The drawing under review shows one solid part. Ordinate dimensions are in mm from its lowest x, y, z. A direction names the side the tool comes from. Round coordinates to 2 decimals unless told otherwise and drop trailing zeros. Order: outer loops, then holes, each group sorted by start corner. A loop starts at its lowest first (then second) coordinate and runs counter-clockwise, first axis right, second up. Notation, with made-up numbers: (88, 43.5) - (124, 43.5) arc R4 ccw to (124, 47.5) - close; hole circle Ø6 at (23, -31). An arc over 180 degrees is marked (long way). One line per question, with ' | ' between items.
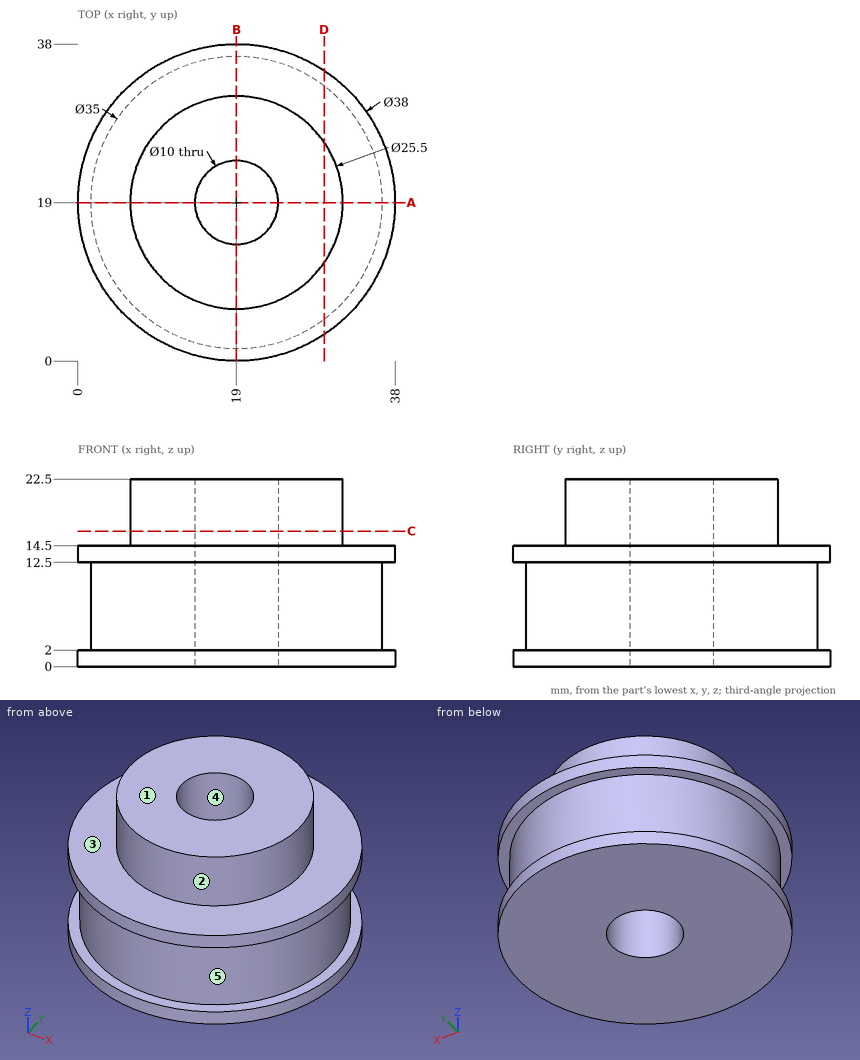
(1) We need section A-A on y = 19. State the section outline as (x, z) points.
Output values:
outline: (0, 0) - (14, 0) - (14, 22.5) - (6.25, 22.5) - (6.25, 14.5) - (0, 14.5) - (0, 12.5) - (1.5, 12.5) - (1.5, 2) - (0, 2) - close; (24, 0) - (38, 0) - (38, 2) - (36.5, 2) - (36.5, 12.5) - (38, 12.5) - (38, 14.5) - (31.75, 14.5) - (31.75, 22.5) - (24, 22.5) - close
(2) Insertion check: pin 1 (8 mm diameter, centred on y = 30, z = 13, fed in from -X); pin 2 (4 mm diameter, centred on x = 28, z = 9.5, fed in from +Y); pin 3 (10 mm diameter, centred on y = 27.5, z = 17.5, fed in from +X); pin 4 (6 mm diameter, centred on x = 19, y = 19, fed in from +Z). Each pin has a flat end and moves straight along its axis. Give the tip position at first contact, or say it passes through.
Output values:
pin 1: x = 1.34 | pin 2: y = 35.04 | pin 3: x = 37.46 | pin 4: through
(3) For probe 1 along Y at (x, z) = (19, 5.75); probe 2 along Z at (x, y) = (13, 2); probe 3 along Y at (x, z) = (19, 13.25), list the stretches that pass through material, from the lowest coordinate up. Write a range as [from, to].
Output values:
probe 1: [1.5, 14], [24, 36.5] | probe 2: [0, 2], [12.5, 14.5] | probe 3: [0, 14], [24, 38]
(4) For the marked faces 1 and 2, list the 3-axis set-ups (+Z, -Z, +X, -X, +Y, -Y) from which the entire face can be reached by the end or side of a thin tool; tool diameter is ignored.
Output values:
face 1: +Z, +X, -X, +Y, -Y | face 2: +Z
(5) We need section C-C on z = 16.25. State the section outline as (x, y) points, plus the area to 3 significant figures.
Output values:
outline: circle Ø25.5 at (19, 19); hole circle Ø10 at (19, 19) | area: 432 mm^2
(6) Mouldability with a two-part tool opening along Z and no side actions: class the marked faces 3, 4 and 5 as released by +Z, released by -Z, zero draft, split by the parting line, or undercut.
Output values:
face 3: released by +Z | face 4: zero draft | face 5: undercut
(7) We need section D-D on x = 29.5. State the section outline as (y, z) points.
Output values:
outline: (3.16, 0) - (34.84, 0) - (34.84, 2) - (33, 2) - (33, 12.5) - (34.84, 12.5) - (34.84, 14.5) - (26.23, 14.5) - (26.23, 22.5) - (11.77, 22.5) - (11.77, 14.5) - (3.16, 14.5) - (3.16, 12.5) - (5, 12.5) - (5, 2) - (3.16, 2) - close
